```python
from build123d import *

# Parameters (mm, degrees)
SKETCH1_W              = 630
SKETCH1_H              = 90
BOSS_EXTRUDE1_DEPTH    = 3
SKETCH3_W              = 30
SKETCH3_H              = 3
CUT_EXTRUDE1_DEPTH     = 3
LPATTERN1_COUNT        = 10
LPATTERN1_PITCH        = 60
LPATTERN1_COL_COUNT    = 2
LPATTERN1_COL_PITCH    = 60
CUT_EXTRUDE5_START     = -3
CUT_EXTRUDE5_OUTLINE_W = 3
CUT_EXTRUDE5_OUTLINE_H = 30
CUT_EXTRUDE5_DEPTH     = 3
SKETCH7_W              = 3
SKETCH7_H              = 30
CUT_EXTRUDE3_DEPTH     = 3
SKETCH13_W             = 3
SKETCH13_H             = 27
CUT_EXTRUDE4_DEPTH     = 10


# Read off the part's stored shape, not the designer's step: Cut-Extrude5
with BuildPart() as part:
    # Sketch1 → Boss-Extrude1 (new body)
    with BuildSketch(Plane(origin=(0, 0, 0), x_dir=(1, 0, 0), z_dir=(0, 1, 0))):
        Rectangle(SKETCH1_W, SKETCH1_H)
    extrude(amount=BOSS_EXTRUDE1_DEPTH)

    # Sketch3 → Cut-Extrude1 (cut)
    with BuildSketch(Plane(origin=(0, 3, 0), x_dir=(1, 0, 0), z_dir=(0, 1, 0))):
        with Locations((-240, -43.5)):
            Rectangle(SKETCH3_W, SKETCH3_H)
    cut_extrude1 = extrude(amount=-CUT_EXTRUDE1_DEPTH, mode=Mode.SUBTRACT)

    # LPattern1: Cut-Extrude1 ×10
    with Locations(*[(i * LPATTERN1_PITCH, 0, 0) for i in range(1, LPATTERN1_COUNT)]):
        add(cut_extrude1, mode=Mode.SUBTRACT)

    # LPattern1 col: Cut-Extrude1 ×2
    with Locations(*[(-i * LPATTERN1_COL_PITCH, 0, 0) for i in range(1, LPATTERN1_COL_COUNT)]):
        add(cut_extrude1, mode=Mode.SUBTRACT)

    # Cut-Extrude5 outline → Cut-Extrude5 (cut)
    with BuildSketch(Plane(origin=(0, 3, 0), x_dir=(1, 0, 0), z_dir=(0, 1, 0)).offset(CUT_EXTRUDE5_START)):
        with Locations((313.5, 1e-09)):
            Rectangle(CUT_EXTRUDE5_OUTLINE_W, CUT_EXTRUDE5_OUTLINE_H)
    extrude(amount=CUT_EXTRUDE5_DEPTH, mode=Mode.SUBTRACT)

    # Sketch7 → Cut-Extrude3 (cut)
    with BuildSketch(Plane(origin=(0, 3, 0), x_dir=(1, 0, 0), z_dir=(0, 1, 0))):
        with Locations((-313.5, 30)):
            Rectangle(SKETCH7_W, SKETCH7_H)
    extrude(amount=-CUT_EXTRUDE3_DEPTH, mode=Mode.SUBTRACT)

    # Sketch13 → Cut-Extrude4 (cut)
    with BuildSketch(Plane(origin=(0, 3, 0), x_dir=(1, 0, 0), z_dir=(0, 1, 0))):
        with Locations((-313.5, -28.5)):
            Rectangle(SKETCH13_W, SKETCH13_H)
    extrude(amount=-CUT_EXTRUDE4_DEPTH, mode=Mode.SUBTRACT)

    # SurfaceCut1
    split(bisect_by=Plane.ZY.offset(-2.6), keep=Keep.BOTTOM)


solid = part.part
```
Geometry: final body of the model. Coordinates: model frame, mm. Give positions to 0.01 mm unless a question says otherwise; leave off trailing zeros. Write each loop counter-clockwise with the first axis right and the second up, starting at its lowest first coordinate (ties: lowest second). Pieces come first, ordered by that corner, then holes.
1. Line query: probe 1 along Z at (x, y) = (58.5, 1.7); probe 2 along X at (y, z) = (2.5, -4). Output: solid intervals per line, ascending.
2. Pin query (flat end, axial travel): P1, Ø1.5, axis at y = 1, z = 43.5, coming from the -X side; P2, Ø0.9, axis at x = 314, y = 1, coming from the +Z side; P3, Ø1.5, axis at y = 1, z = 43, coming from the +X side. Return the tip coordinate at first contact, or that it passes through.
3. Section query A-A, the plane y = 0.95. Return loops of the section in (x, z), then the cut area to 3 significant figures.
4. Section query B-B, the plane x = 58.5. Return loops of the section in (y, z), then the cut area to 3 significant figures.
Computed:
1. probe 1: z = -45 to 42
1. probe 2: x = 2.6 to 312
2. P1: stops at x = 15
2. P2: stops at z = 42
2. P3: stops at x = 285
3. outline: (2.6, -45) - (315, -45) - (315, -15) - (312, -15) - (312, 15) - (315, 15) - (315, 42) - (285, 42) - (285, 45) - (255, 45) - (255, 42) - (225, 42) - (225, 45) - (195, 45) - (195, 42) - (165, 42) - (165, 45) - (135, 45) - (135, 42) - (105, 42) - (105, 45) - (75, 45) - (75, 42) - (45, 42) - (45, 45) - (15, 45) - (15, 42) - (2.6, 42) - close
3. area: 27,500 mm2
4. outline: (0, -45) - (3, -45) - (3, 42) - (0, 42) - close
4. area: 261 mm2
